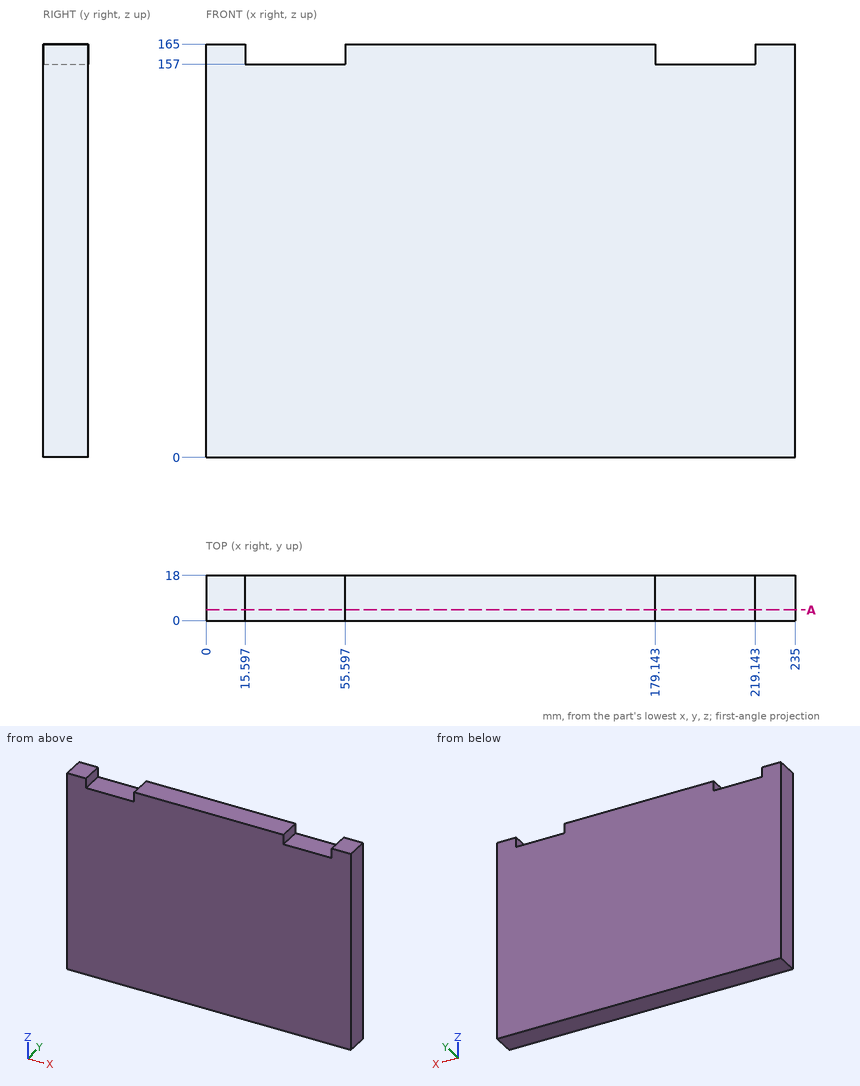
Print and shaded views of the part. All mm, measured from the part's lowest x, y and z. Coordinates: 2 decimals unless noted, no trailing zeros. Write each loop counter-clockwise with the first axis right and the second up, starting at its lowest first coordinate (ties: lowest second). Pieces come first, ordered by that corner, then holes. Notation, with made-up numbers: M 34,0.25 L 87,0.25 A20 ccw 87,26.25 Z; hole C 31,-39.5 d8. An arc over 180 degrees is marked long. Return JSON: item names as keys, results as strings.
1. Saw through at A-A, the plane y = 4.25. Write the cut outline in (x, z), then the cut area to 3 significant figures.
Determined:
{"outline": "M 0,0 L 235,0 L 235,165 L 219.14,165 L 219.14,157 L 179.14,157 L 179.14,165 L 55.6,165 L 55.6,157 L 15.6,157 L 15.6,165 L 0,165 Z", "area": "38,100 mm²"}
2. Probe L1, parallel to X at y = 16, z = 157.5; L2, parallel to Z at x = 49.5, y = 8. List the from-to ranges inside material, lowest first.
Determined:
{"L1": "0 to 15.6, 55.6 to 179.14, 219.14 to 235", "L2": "0 to 157"}
3. Flat gauge pins, fed straight in: pin 1 Ø3 at (x, y) = (38.5, 10) entering from +Z; pin 2 Ø10 at (x, z) = (136.5, 112) entering from -Y. Where does each tip first touch, or does it go through?
Determined:
{"pin 1": "z = 157", "pin 2": "y = 0"}
